Input: dimensioned drawing with shaded views. Units: mm. Origin: part minimum x, y, z. A direction names the side the tool comes from. Round coordinates to 2 decimals unless told otherwise and drop trailing zeros. Order: outer loops, then holes, each group sorted by start corner. A loop starts at its lowest first (then second) coordinate and runs counter-clockwise, first axis right, second up. Notation, with made-up numbers: M 73.25,-37.75 L 125.25,-37.75 A19 ccw 125.25,-8.75 Z; hole C 66.5,-3 d1. An arc over 180 degrees is marked long. Use one line per item in the form item = value. Start each with the question number.
Q1. Section A-A (y = 19). Return the cut outline in (x, z), plus the area to 3 significant figures.
Q2. Reachability of the marked faces 4 and 5 from +Z, -Z, +X, -X, +Y, -Y: full face, straight path, thin tool, end or side. Return the list, or none.
Q3. Material intervals for probe 1 along Z at (x, y) = (127.5, 6.5); probe 2 along Y at (x, z) = (179, 184); probe 3 along Z at (x, y) = (191, 38), sorted ascending.
Q4. Pull-direction query (Z, two-part tool) for the marked faces 1, 2 and 3; classes: pulls with the +Z half, pulls with the -Z half, needs draft (parallel to the pull), parting line crosses it, or undercut.
Q5. Section D-D (z = 208.5). Return the cut outline in (x, y), plus the area to 3 significant figures.
Q6. Contact query for flat-ended pins moving along their axis: pin 1 (5 mm diameter, centred on y = 8, z = 243.5, fed in from +X); pin 2 (5 mm diameter, centred on x = 181.5, z = 213, fed in from -Y). Output: stop coordinate, or through.
Q7. Section B-B (x = 20). Return the cut outline in (y, z), plus the area to 3 significant figures.
Q8. Section C-C (z = 117.5). Return the cut outline in (x, y), plus the area to 3 significant figures.
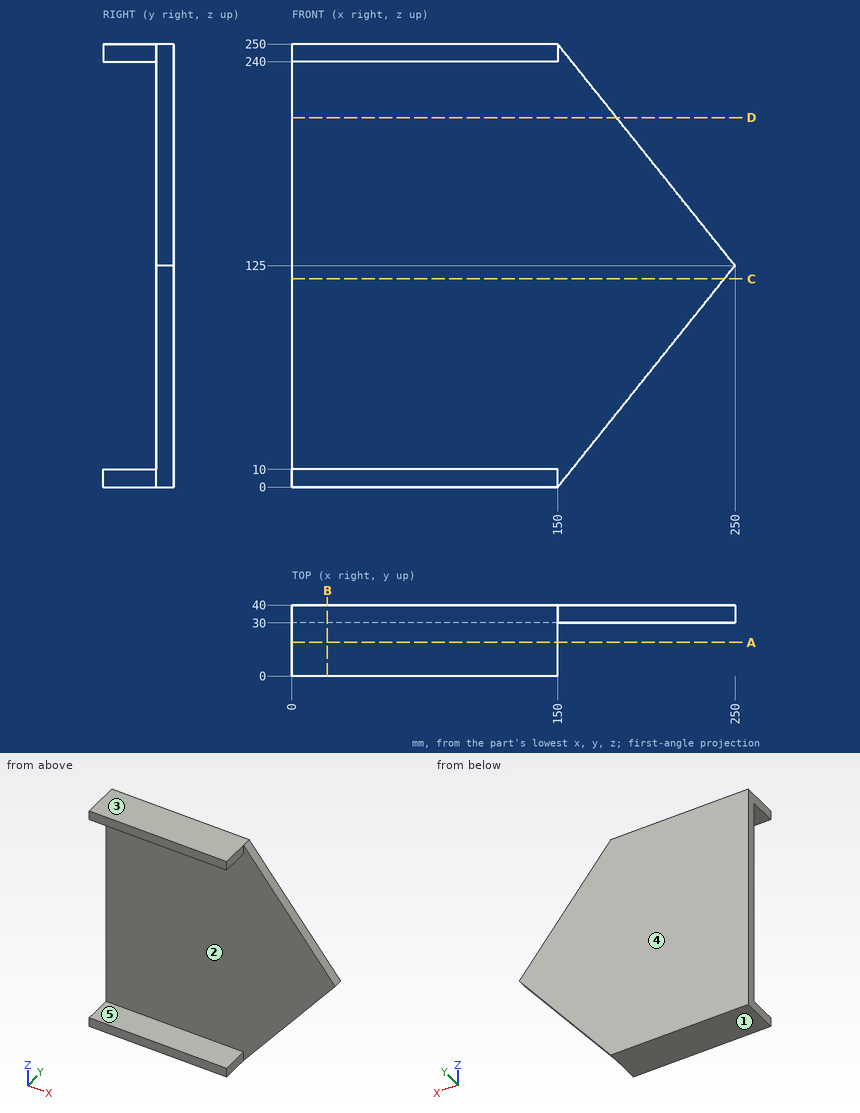
Results list:
q1.outline = M 0,0 L 150,0 L 150,10 L 0,10 Z; M 0,240 L 150,240 L 150,250 L 0,250 Z
q1.area = 3,000 mm2
q2.face_4 = +Z, -Z, +X, -X, +Y
q2.face_5 = +X, -X, -Y
q3.probe_1 = 0 to 10, 240 to 250
q3.probe_2 = 30 to 40
q3.probe_3 = 51.25 to 198.75
q4.face_1 = pulls with the -Z half
q4.face_2 = undercut
q4.face_3 = pulls with the +Z half
q5.outline = M 0,30 L 183.2,30 L 183.2,40 L 0,40 Z
q5.area = 1,830 mm2
q6.pin_1 = 150
q6.pin_2 = 30
q7.outline = M 0,0 L 40,0 L 40,250 L 0,250 L 0,240 L 30,240 L 30,10 L 0,10 Z
q7.area = 3,100 mm2
q8.outline = M 0,30 L 244,30 L 244,40 L 0,40 Z
q8.area = 2,440 mm2
